from build123d import *

# Parameters (mm, degrees)
F1_DEPTH = 1.2
F2_R     = 3.5
F3_DEPTH = 1.2
F4_R     = 1.55
F5_DEPTH = 2.4


with BuildPart() as f1:
    # F0 (on Top) → F1 (new body)
    with BuildSketch(Plane.XY):
        with BuildLine():
            Line((59.5437594947, 4.4768118791), (-59.5437594947, 4.4768118791))
            ThreePointArc((-59.5437594947, 4.4768118791), (-64.494199231, 0.2284146929), (-60, -4.5))
            Line((-60, -4.5), (60, -4.5))
            ThreePointArc((60, -4.5), (64.494199231, 0.2284146929), (59.5437594947, 4.4768118791))
        make_face()
    extrude(amount=F1_DEPTH)

    # F2 (on face) → F3 (join)
    with BuildSketch(Plane.XY):
        with Locations((-60, 0)):
            Circle(F2_R)
        Circle(F2_R)
        with Locations((60, 0)):
            Circle(F2_R)
    extrude(amount=-F3_DEPTH)

    # F4 (on face) → F5 (cut, through all)
    with BuildSketch(Plane(origin=(0, 0, -1.2), x_dir=(1, 0, 0), z_dir=(0, 0, -1))):
        with Locations((60, 0)):
            Circle(F4_R)
        Circle(F4_R)
        with Locations((-60, 0)):
            Circle(F4_R)
    extrude(amount=-F5_DEPTH, mode=Mode.SUBTRACT)


solid = f1.part
Can you work these out from the model? Positions are in its coordinate system, mm. A direction names the side the tool comes from. Give positions to 0.01 mm unless a question says otherwise; leave off trailing zeros. Loops run counter-clockwise (first coordinate to the right, second up) from the corner with the lowest first, then second, coordinate; pieces in that order, holes last. Notation, with made-up numbers: (62, 38) -> (68, 38) arc R32 ccw to (68, 72) -> close; hole circle Ø11 at (-2, -16.5). An arc over 180 degrees is marked (long way). Return JSON: item names as keys, results as strings.
Q1. I want a section at A-A, the plane x = 0. List the corners of the cut face in (y, z) for me, then the cut area to 3 significant figures.
Checks:
{"outline": "(-4.5, 0) -> (-3.5, 0) -> (-3.5, -1.2) -> (-1.55, -1.2) -> (-1.55, 1.2) -> (-4.5, 1.2) -> close; (1.55, -1.2) -> (3.5, -1.2) -> (3.5, 0) -> (4.48, 0) -> (4.48, 1.2) -> (1.55, 1.2) -> close", "area": "11.7 mm2"}
Q2. I want a section at C-C, the plane z = 0.75. List the corners of the cut face in (x, y) for me, then the cut area to 3 significant figures.
Checks:
{"outline": "(-60, -4.5) -> (60, -4.5) arc R4.5 ccw (long way) to (59.54, 4.48) -> (-59.54, 4.48) arc R4.5 ccw (long way) to start; hole circle Ø3.1 at (-60, 0); hole circle Ø3.1 at (0, 0); hole circle Ø3.1 at (60, 0)", "area": "1,120 mm2"}
Q3. I want a section at D-D, the plane x = -21.5. List the corners of the cut face in (y, z) for me, then the cut area to 3 significant figures.
Checks:
{"outline": "(-4.5, 0) -> (4.48, 0) -> (4.48, 1.2) -> (-4.5, 1.2) -> close", "area": "10.8 mm2"}
Q4. I need wall thicknesses on probe 1 along X at (y, z) = (0, 0.7); probe 2 along X at (y, z) = (0.25, -0.7); probe 3 along X at (y, z) = (3, -0.4). Which ranges of each line are inside material? Lowest first, please.
Checks:
{"probe 1": "x = -64.5 to -61.55, -58.45 to -1.55, 1.55 to 58.45, 61.55 to 64.5", "probe 2": "x = -63.49 to -61.53, -58.47 to -56.51, -3.49 to -1.53, 1.53 to 3.49, 56.51 to 58.47, 61.53 to 63.49", "probe 3": "x = -61.8 to -58.2, -1.8 to 1.8, 58.2 to 61.8"}
Q5. For pin 1 Ø0.6 at (x, z) = (1, 0.5) entering from +Y; pin 2 Ø1 at (x, y) = (21, 2.5) entering from -Z, each with a flat end and sliding along its axis, tell me the tip position at first contact or that it passes through.
Checks:
{"pin 1": "stops at y = 4.48", "pin 2": "stops at z = 0"}
Q6. We'd pull the mould along Y, two halves only. Please class faces 3 (the face through (3.233, -1.341, -0.592)), 4 (the face through (0.715, 1.375, -0.017)), 5 (the face through (62, -1, -1.2)): released by +Y, released by -Y, zero draft, split by the parting line, or undercut.
Checks:
{"face 3": "split by the parting line", "face 4": "undercut", "face 5": "zero draft"}
Q7. I want a section at B-B, the plane y = 0. List the corners of the cut face in (x, z) for me, then the cut area to 3 significant figures.
Checks:
{"outline": "(-64.5, 0) -> (-63.5, 0) -> (-63.5, -1.2) -> (-61.55, -1.2) -> (-61.55, 1.2) -> (-64.5, 1.2) -> close; (-58.45, -1.2) -> (-56.5, -1.2) -> (-56.5, 0) -> (-3.5, 0) -> (-3.5, -1.2) -> (-1.55, -1.2) -> (-1.55, 1.2) -> (-58.45, 1.2) -> close; (1.55, -1.2) -> (3.5, -1.2) -> (3.5, 0) -> (56.5, 0) -> (56.5, -1.2) -> (58.45, -1.2) -> (58.45, 1.2) -> (1.55, 1.2) -> close; (61.55, -1.2) -> (63.5, -1.2) -> (63.5, 0) -> (64.5, 0) -> (64.5, 1.2) -> (61.55, 1.2) -> close", "area": "158 mm2"}
Q8. On a 3-axis mill with a long thin cutter (end or side, diameter ignored), from which of +Z, -Z, +X, -X, +Y, -Y can I reach the whole of each face in a straight line? I mean faces 1 (the face through (-1, -2, 1.2)), 2 (the face through (56.503, 0.154, -0.592)). Say none if no direction works.
Checks:
{"face 1": "+Z, +X, -X, +Y, -Y", "face 2": "-Z"}
